```python
from build123d import *

# Parameters (mm, degrees)
SKETCH1_R                    = 3.175
BOSS_EXTRUDE1_DEPTH          = 3.175
F_1_8_0_125_DIAMETER_HOLE1_D = 3.175


with BuildPart() as part:
    # Sketch1 → Boss-Extrude1 (new body)
    with BuildSketch(Plane.XY):
        with BuildLine():
            Line((-8.682173031, 0.326637814), (-2.477735609, 25.4))
            ThreePointArc((-2.477735609, 25.4), (-0.013242247, 27.329875409), (2.45298258, 25.402213164))
            Line((2.45298258, 25.402213164), (8.681575809, 0.327789055))
            ThreePointArc((8.681575809, 0.327789055), (8.744087205, -0.033833939), (8.753834359, -0.400690665))
            ThreePointArc((8.753834359, -0.400690665), (-0.00074846, -8.762999968), (-8.753902679, -0.399195305))
            ThreePointArc((-8.753902679, -0.399195305), (-8.744226674, -0.033690664), (-8.682173031, 0.326637814))
        make_face()
        Circle(SKETCH1_R, mode=Mode.SUBTRACT)
    extrude(amount=BOSS_EXTRUDE1_DEPTH)

    # 1/8 (0.125) Diameter Hole1 (through all)
    with Locations(Plane.XY.offset(3.175)):
        with Locations((0, 17.804875409)):
            Hole(F_1_8_0_125_DIAMETER_HOLE1_D / 2)


solid = part.part
```
Verification items for the finished model (mm, model axes). Coordinates: 2 decimals unless noted, no trailing zeros. Loops run counter-clockwise (first coordinate to the right, second up) from the corner with the lowest first, then second, coordinate; pieces in that order, holes last. Notation, with made-up numbers: (-32.5, 29) -> (-22.5, 29) arc R23 ccw to (-22.5, 62) -> close; hole circle Ø1 at (83.25, -21.5). An arc over 180 degrees is marked (long way). Put each result on its own line as item: value.
1. Section check A-A, the plane x = -0.75. Record the boundary of the cut face in (y, z) (3 decimals).
Result set:
outline: (-8.731, 0) -> (-3.085, 0) -> (-3.085, 3.175) -> (-8.731, 3.175) -> close; (3.085, 0) -> (16.406, 0) -> (16.406, 3.175) -> (3.085, 3.175) -> close; (19.204, 0) -> (27.22, 0) -> (27.22, 3.175) -> (19.204, 3.175) -> close
2. Section check B-B, the plane y = 0. Record the boundary of the cut face in (x, z) (1 decimal).
Result set:
outline: (-8.7, 0) -> (-3.2, 0) -> (-3.2, 3.2) -> (-8.7, 3.2) -> close; (3.2, 0) -> (8.7, 0) -> (8.7, 3.2) -> (3.2, 3.2) -> close
3. Section check D-D, the plane y = -5.5. Record the boundary of the cut face in (x, z) (3 decimals).
Result set:
outline: (-6.822, 0) -> (6.822, 0) -> (6.822, 3.175) -> (-6.822, 3.175) -> close
4. Thickness scan on line 1 (Y direction, x = 0, z = 1.2) (3 decimals); line 2 (X direction, y = 19, z = 0.25); line 3 (X direction, y = 2.5, z = 1.05). Record the ranges inside material, lowest first.
Result set:
line 1: y = -8.763 to -3.175, 3.175 to 16.217, 19.392 to 27.33
line 2: x = -4.06 to -1.04, 1.04 to 4.04
line 3: x = -8.14 to -1.96, 1.96 to 8.14
5. Gauge pin test, flat ends, axial feed: P1, Ø1, axis at y = 10.5, z = 2.5, coming from the +X side; P2, Ø1.5, axis at y = 22.5, z = 0.5, coming from the +X side. Record the tip position at first contact, or that the pin passes through.
Result set:
P1: stops at x = 6.28
P2: stops at x = 3.36
6. Section check C-C, the plane x = 4.5. Record the boundary of the cut face in (y, z) (3 decimals).
Result set:
outline: (-7.519, 0) -> (17.162, 0) -> (17.162, 3.175) -> (-7.519, 3.175) -> close
7. Mould release check, pull along X, two halves, no side actions. Record for faces 1 (the face through (0, 6, 0)), 2 (the face through (-0.69, -3.1, 1.57)), 3 (the face through (5.524, 13.041, 1.565)), 4 (the face through (-5.623, 12.688, 1.565)): pulls with the +X half, pulls with the -X half, needs draft (parallel to the pull), parting line crosses it, or undercut.
Result set:
face 1: needs draft
face 2: undercut
face 3: pulls with the +X half
face 4: pulls with the -X half
